Geometry check sheet. Reference: the model listing, model coordinates, mm. A direction names the side the tool comes from. Give positions to 0.01 mm unless a question says otherwise; leave off trailing zeros. Order: outer loops, then holes, each group sorted by start corner. A loop starts at its lowest first (then second) coordinate and runs counter-clockwise, first axis right, second up.
from build123d import *

# Parameters (mm, degrees)
BOSS_EXTRUDE1_DEPTH = 20
SKETCH2_R           = 6
CUT_EXTRUDE1_DEPTH  = 4
SKETCH3_R           = 1.5
CUT_EXTRUDE2_DEPTH  = 4
FILLET1_R           = 2


with BuildPart() as part:
    # Sketch1 → Boss-Extrude1 (new body)
    with BuildSketch(Plane.XY):
        Polygon((0, 0), (23, 0), (23, 4), (4, 4), (4, 34), (0, 34), align=None)
    extrude(amount=BOSS_EXTRUDE1_DEPTH)

    # Sketch2 → Cut-Extrude1 (cut)
    with BuildSketch(Plane.ZY):
        with Locations((10, 24)):
            Circle(SKETCH2_R)
    extrude(amount=-CUT_EXTRUDE1_DEPTH, mode=Mode.SUBTRACT)

    # Sketch3 → Cut-Extrude2 (cut)
    with BuildSketch(Plane(origin=(0, 4, 0), x_dir=(1, 0, 0), z_dir=(0, 1, 0))):
        with Locations((18, -10)):
            Circle(SKETCH3_R)
        with Locations((10, -10)):
            Circle(SKETCH3_R)
    extrude(amount=-CUT_EXTRUDE2_DEPTH, mode=Mode.SUBTRACT)

    # Fillet1
    fillet1_edges = [part.edges().sort_by_distance(p)[0] for p in [
        (23, 2, 20),
        (4, 4, 10),
        (0, 0, 10),
        (2, 34, 20),
        (2, 34, 0),
        (23, 2, 0),
    ]]
    fillet(fillet1_edges, radius=FILLET1_R)


solid = part.part
Item 1: Sectioned sample at D-D (z = 8). Enter the section's corners in (x, y).
Reported:
outline: (0, 2) arc R2 ccw to (2, 0) - (23, 0) - (23, 4) - (6, 4) arc R2 cw to (4, 6) - (4, 18.34) - (0, 18.34) - close; (0, 29.66) - (4, 29.66) - (4, 34) - (0, 34) - close
Item 2: Sectioned sample at B-B (z = 3). Enter the section's corners in (x, y).
Reported:
outline: (0, 2) arc R2 ccw to (2, 0) - (23, 0) - (23, 4) - (6, 4) arc R2 cw to (4, 6) - (4, 34) - (0, 34) - close
Item 3: Draft check along X on faces 1 (the flat face through (15, 4, 10)), 2 (the cylindrical face through (4.6, 4.57, 10.14)), 3 (the cylindrical face through (16.5, 2.03, 9.93)). Enter one of: released by +X, released by -X, zero draft, split by the parting line, or undercut.
Reported:
face 1: zero draft
face 2: released by +X
face 3: undercut
Item 4: Sectioned sample at A-A (x = 18). Enter the section's corners in (y, z), and give its area (3 significant figures).
Reported:
outline: (0, 0) - (4, 0) - (4, 8.5) - (0, 8.5) - close; (0, 11.5) - (4, 11.5) - (4, 20) - (0, 20) - close
area: 68.0 mm2
Item 5: Scan lines: L1, parallel to Y at x = 3.05, z = 10; L2, parallel to Z at x = 18, y = 0.8; L3, parallel to X at y = 20, z = 3.5. Record each from-to range of solid material in increasing order.
Reported:
L1: y = 0 to 18, 30 to 34
L2: z = 0 to 8.5, 11.5 to 20
L3: x = 0 to 4
Item 6: Sectioned sample at C-C (y = 24). Enter the section's corners in (x, z).
Reported:
outline: (0, 0) - (4, 0) - (4, 4) - (0, 4) - close; (0, 16) - (4, 16) - (4, 20) - (0, 20) - close
Item 7: Gauge pin test, flat ends, axial feed: pin 1 (4 mm diameter, centred on x = 15.5, z = 9, fed in from +Y); pin 2 (5 mm diameter, centred on x = 19.5, z = 10.5, fed in from -Y); pin 3 (2 mm diameter, centred on y = 30.5, z = 7, fed in from +X). Record the tip position at first contact, or that the pin passes through.
Reported:
pin 1: stops at y = 4
pin 2: stops at y = 0
pin 3: stops at x = 4
Item 8: Set-up check for faces 4 (the cylindrical face through (22.4, 2.03, 19.43)), 5 (the flat face through (4, 17, 10)): record each of +Z, -Z, +X, -X, +Y, -Y from which the full face is reachable in a straight line by a thin tool's end or side.
Reported:
face 4: +Z, +X, +Y, -Y
face 5: +Z, -Z, +X, +Y
